Verification items for the finished model (mm, model axes). Give positions to 0.01 mm unless a question says otherwise; leave off trailing zeros. Loops run counter-clockwise (first coordinate to the right, second up) from the corner with the lowest first, then second, coordinate; pieces in that order, holes last. Notation, with made-up numbers: (75.25, 21) - (80.25, 21) arc R11 cw to (80.25, 27) - close; hole circle Ø7 at (-29, 29). An arc over 180 degrees is marked (long way). Use one line per item in the form item = value.
```python
from build123d import *

# Parameters (mm, degrees)
CROQUIS1_W              = 230
CROQUIS1_H              = 230
SALIENTE_EXTRUIR1_DEPTH = 3
REDONDEO1_R             = 30
REDONDEO2_R             = 30
REDONDEO3_R             = 30
REDONDEO4_R             = 30
CROQUIS2_R              = 1.5
CORTAR_EXTRUIR1_DEPTH   = 3


with BuildPart() as part:
    # Croquis1 → Saliente-Extruir1 (new body)
    with BuildSketch(Plane.XY):
        Rectangle(CROQUIS1_W, CROQUIS1_H)
    extrude(amount=SALIENTE_EXTRUIR1_DEPTH)

    # Redondeo1
    redondeo1_edges = [part.edges().sort_by_distance(p)[0] for p in [
        (115, 115, 1.5),
    ]]
    fillet(redondeo1_edges, radius=REDONDEO1_R)

    # Redondeo2
    redondeo2_edges = [part.edges().sort_by_distance(p)[0] for p in [
        (115, -115, 1.5),
    ]]
    fillet(redondeo2_edges, radius=REDONDEO2_R)

    # Redondeo3
    redondeo3_edges = [part.edges().sort_by_distance(p)[0] for p in [
        (-115, -115, 1.5),
    ]]
    fillet(redondeo3_edges, radius=REDONDEO3_R)

    # Redondeo4
    redondeo4_edges = [part.edges().sort_by_distance(p)[0] for p in [
        (-115, 115, 1.5),
    ]]
    fillet(redondeo4_edges, radius=REDONDEO4_R)

    # Croquis2 → Cortar-Extruir1 (cut)
    with BuildSketch(Plane.XY.offset(3)):
        with Locations((-70.125, 69.25)):
            Circle(CROQUIS2_R)
        with Locations((-70.125, 46.75)):
            Circle(CROQUIS2_R)
        with Locations((-22.875, 46.75)):
            Circle(CROQUIS2_R)
        with Locations((22.875, 69.25)):
            Circle(CROQUIS2_R)
        with Locations((22.875, 46.75)):
            Circle(CROQUIS2_R)
        with Locations((70.125, 46.75)):
            Circle(CROQUIS2_R)
        with Locations((70.125, 69.25)):
            Circle(CROQUIS2_R)
        with Locations((70.125, -69.25)):
            Circle(CROQUIS2_R)
        with Locations((70.125, -46.75)):
            Circle(CROQUIS2_R)
        with Locations((22.875, -46.75)):
            Circle(CROQUIS2_R)
        with Locations((22.875, -69.25)):
            Circle(CROQUIS2_R)
        with Locations((-22.875, -69.25)):
            Circle(CROQUIS2_R)
        with Locations((-70.125, -69.25)):
            Circle(CROQUIS2_R)
        with Locations((-70.125, -46.75)):
            Circle(CROQUIS2_R)
        with Locations((-22.875, -46.75)):
            Circle(CROQUIS2_R)
        with Locations(Location((-22.875, 69.25, 0), (0, 0, 180))):
            Circle(CROQUIS2_R)
    extrude(amount=-CORTAR_EXTRUIR1_DEPTH, mode=Mode.SUBTRACT)


solid = part.part
```
1. Section check A-A, the plane z = 0.55. State how many separate pieces and enclosed holes the cut face has, then the cut area to 3 significant figures.
Result set:
separate_pieces = 1
enclosed_holes = 16
area = 52,000 mm²
2. Section check B-B, the plane x = -96.5. Record the cut outline in (y, z).
Result set:
outline = (-112.71, 0) - (112.71, 0) - (112.71, 3) - (-112.71, 3) - close
3. Scan lines: probe 1 along X at (y, z) = (69.25, 1.9) (3 decimals); probe 2 along Y at (x, z) = (71, 2.8); probe 3 along Y at (x, z) = (-105.5, 0.9). Record each from-to range of solid material in increasing order.
Result set:
probe_1 = -115 to -71.625, -68.625 to -24.375, -21.375 to 21.375, 24.375 to 68.625, 71.625 to 115
probe_2 = -115 to -70.47, -68.03 to -47.97, -45.53 to 45.53, 47.97 to 68.03, 70.47 to 115
probe_3 = -106.9 to 106.9
4. Depth check by flat-ended pin: pin 1 Ø1.8 at (x, y) = (70.125, -46.75) entering from -Z; pin 2 Ø4 at (x, y) = (-22.875, 46.75) entering from -Z. Enter the tip coordinate at first touch or a pass-through.
Result set:
pin_1 = through
pin_2 = 0
